Here's how the part is built. I have some questions about the finished solid (model axes, mm). Face numbers are marked on the shaded views. A direction names the side the tool comes from. Give positions to 0.01 mm unless a question says otherwise; leave off trailing zeros. Write each loop counter-clockwise with the first axis right and the second up, starting at its lowest first coordinate (ties: lowest second). Pieces come first, ordered by that corner, then holes. Notation, with made-up numbers: (10.5, -1) - (62.5, -1) arc R26 ccw to (62.5, 38) - close; hole circle Ø3 at (1.5, 85). An arc over 180 degrees is marked (long way). Write each question's results on one line, items separated by ' | '. Start each with the question number.
Item 1: Suppose I cut it at C-C on x = 0. List the corners of the cut face in (y, z) for me, then the cut area to 3 significant figures.
Item 2: We'd pull the mould along X, two halves only. Please class the marked faces 1, 2, 3 and 4: +X half, -X half, draft (parallel to the pull), parting line (faces both ways), or undercut.
Item 3: Will these pins go through, and if not, where does the flat tip stop? P1, Ø2, axis at x = -22.5, y = 21.5, coming from the -Z side; P2, Ø7.5, axis at x = 0, y = 0, coming from the +Z side; P3, Ø3, axis at x = 32.5, z = 7.5, coming from the -Y side; P4, Ø6, axis at y = 22.5, z = 9, coming from the +X side.
Item 4: Which directions (+Z, -Z, +X, -X, +Y, -Y) give clear straight access to the entire face, cutting with the end or side of a thin tool? Please do the marked faces 5 and 6.
Item 5: Suppose I cut it at A-A on z = 1. List the corners of the cut face in (x, y) for me.
Item 6: Suppose I cut it at D-D on x = -31. List the corners of the cut face in (y, z) for me.
Item 7: Suppose I cut it at B-B on y = 0. List the corners of the cut face in (x, z) for me.
Item 8: Please list where these lines run through material, in increasing order: line 1 along Z through (x, y) = (-34, 21.5); line 2 along X through (y, z) = (-33.5, 2); line 3 along X through (y, z) = (13, 2).
```python
from build123d import *

# Parameters (mm, degrees)
F4_T           = -3
F5_D           = 12.5
F5_DEPTH       = 5
F5_START       = 11
F5_CSINK_D     = 14
F5_CSINK_ANGLE = 90
F5_TIP         = 3.7553788689


with BuildPart() as f2:
    # F2: sweep along a path in F1
    with BuildLine(Plane.XZ) as f2_path:
        Line((0, 0), (0, 14))
    # F0 (on Top) → F2 (sweep)
    with BuildSketch(Plane.XY):
        Polygon((2.618910053, -46.1880215352), (41.3094550265, -20.8259681314), (38.6905449735, 25.3620534037), (-2.618910053, 46.1880215352), (-41.3094550265, 20.8259681314), (-38.6905449735, -25.3620534037), align=None)
    sweep(path=f2_path.line)

    # F4
    f4_openings = [f2.faces().sort_by_distance(p)[0] for p in [
        (0, 0, 0),
    ]]
    offset(amount=F4_T, openings=f4_openings)

    # F5
    # its depths count from where the whole tool has entered the part; down to there all is cleared
    with Locations(Plane(origin=(0, 0, 0), x_dir=(1, 0, 0), z_dir=(0, 0, -1))):
        with Locations((0, 0)):
            Hole(F5_CSINK_D / 2, depth=F5_START)
    with Locations(Plane(origin=(0, 0, 0), x_dir=(1, 0, 0), z_dir=(0, 0, -1)).offset(-F5_START)):
        with Locations((0, 0)):
            CounterSinkHole(F5_D / 2, F5_CSINK_D / 2, depth=F5_DEPTH, counter_sink_angle=F5_CSINK_ANGLE)
            with Locations((0, 0, -(F5_DEPTH + F5_TIP / 2))):  # 118° drill point
                Cone(0, F5_D / 2, F5_TIP, mode=Mode.SUBTRACT)


solid = f2.part
```
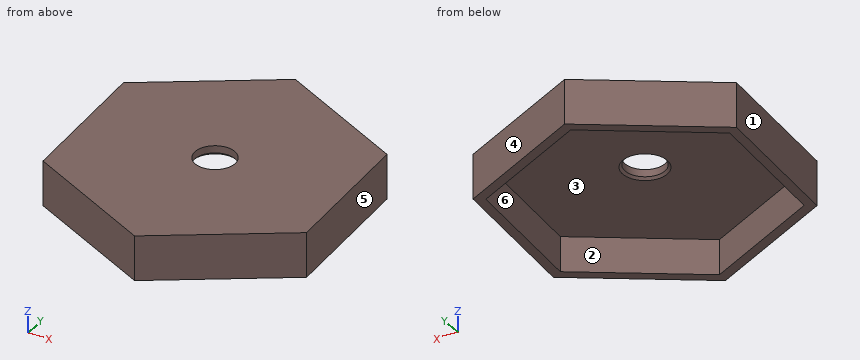
Checked values:
1) outline: (-44.87, 0) - (-41.51, 0) - (-41.51, 11) - (-7, 11) - (-6.25, 11.75) - (-6.25, 14) - (-44.87, 14) - close; (6.25, 11.75) - (7, 11) - (41.51, 11) - (41.51, 0) - (44.87, 0) - (44.87, 14) - (6.25, 14) - close | area: 305 mm^2
2) face 1: -X half | face 2: undercut | face 3: undercut | face 4: +X half
3) P1: stops at z = 11 | P2: passes through | P3: stops at y = -27.58 | P4: stops at x = 39.02
4) face 5: +Z, -Z, +X, +Y | face 6: -Z
5) outline: (-41.31, 20.83) - (-38.69, -25.36) - (2.62, -46.19) - (41.31, -20.83) - (38.69, 25.36) - (-2.62, 46.19) - close; hole (-38.22, 19.27) - (-35.79, -23.46) - (2.42, -42.73) - (38.22, -19.27) - (35.79, 23.46) - (-2.42, 42.73) - close
6) outline: (-29.24, 0) - (-25.88, 0) - (-25.88, 11) - (24, 11) - (24, 0) - (27.58, 0) - (27.58, 14) - (-29.24, 14) - close
7) outline: (-40.13, 0) - (-37.12, 0) - (-37.12, 11) - (-7, 11) - (-6.25, 11.75) - (-6.25, 14) - (-40.13, 14) - close; (6.25, 11.75) - (7, 11) - (37.12, 11) - (37.12, 0) - (40.13, 0) - (40.13, 14) - (6.25, 14) - close
8) line 1: z = 11 to 14 | line 2: x = -22.55 to -15.88, 16.5 to 21.97 | line 3: x = -40.87 to -37.86, 36.39 to 39.39
